Check sheet for the drawn part. Datum: minimum x, y, z corner. Units: mm. Give positions to 0.01 mm unless a question says otherwise; leave off trailing zeros. Order: outer loops, then holes, each group sorted by start corner. A loop starts at its lowest first (then second) coordinate and runs counter-clockwise, first axis right, second up. Notation, with made-up numbers: (-39, 1) -> (-8, 1) arc R18 ccw to (-8, 24) -> close; hole circle Ø4 at (34.5, -38.5). An arc over 180 degrees is marked (long way). Return JSON: item names as keys, results as strings. Group by question number.
(1) Cross-section at A-A on x = 4.5. Enter the section's corners in (y, z).
(2) Thickness scan on line 1 along X through (y, z) = (3.45, 0.7); line 2 along Y through (x, z) = (3.45, 0.5); line 3 along X through (y, z) = (4.25, 0.75) (1 decimal). Record the ranges inside material, lowest first.
(3) Cross-section at C-C on z = 0.75. Enter the section's corners in (x, y).
(4) Cross-section at D-D on x = 1.25. Enter the section's corners in (y, z).
(5) Cross-section at B-B on y = 2.5. Enter the section's corners in (x, z).
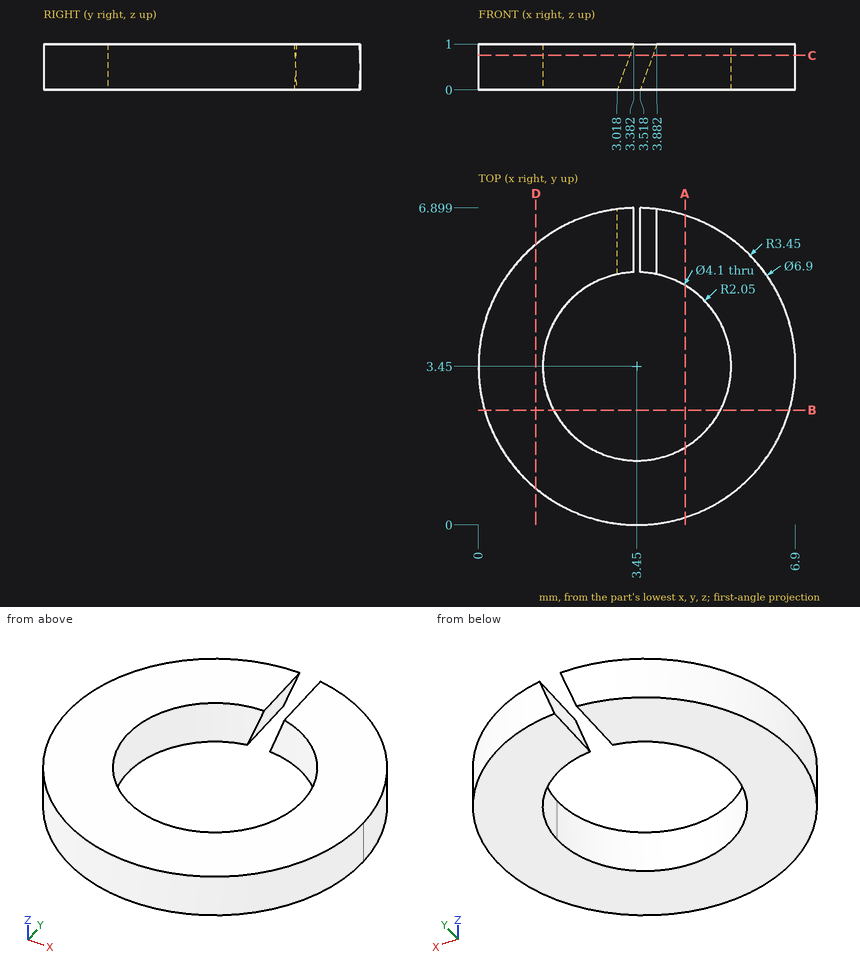
Verdict:
{
 "1": {"outline": "(0.16, 0) -> (1.69, 0) -> (1.69, 1) -> (0.16, 1) -> close; (5.21, 0) -> (6.74, 0) -> (6.74, 1) -> (5.21, 1) -> close"},
 "2": {"line 1": "0 to 1.4, 5.5 to 6.9", "line 2": "0 to 1.4", "line 3": "0.1 to 1.6, 5.3 to 6.8"},
 "3": {"outline": "(3.29, 5.49) -> (3.29, 6.9) arc R3.45 ccw (long way) to (3.79, 6.88) -> (3.79, 5.47) arc R2.05 cw (long way) to start"},
 "4": {"outline": "(0.79, 0) -> (6.11, 0) -> (6.11, 1) -> (0.79, 1) -> close"},
 "5": {"outline": "(0.13, 0) -> (1.63, 0) -> (1.63, 1) -> (0.13, 1) -> close; (5.27, 0) -> (6.77, 0) -> (6.77, 1) -> (5.27, 1) -> close"}
}
